Geometry: final body of the model. Coordinates: model frame, mm. Give positions to 0.01 mm unless a question says otherwise; leave off trailing zeros. Write each loop counter-clockwise with the first axis right and the second up, starting at its lowest first coordinate (ties: lowest second). Pieces come first, ordered by that corner, then holes. Notation, with made-up numbers: M 71,32 L 75,32 A11 ccw 75,49 Z; hole C 14.25,66 d3. An arc over 180 degrees is marked long. Use a Markdown table: item, result. Add a question column.
(1) Draft query along X for faces 1 (the flat face through (36, 0, -3)), 2 (the flat face through (0, 3, -3)), 3 (the cylindrical face through (1.735, 2.958, -2.194)). Return one class per face: released by +X, released by -X, zero draft, split by the parting line, or undercut.
(2) Material intervals for L1, parallel to Y at x = 9, z = -3.4; L2, parallel to Z at x = 3, y = 2.7; L3, parallel to X at y = 3, z = -3.8, sorted ascending.
(3) Cut plane A-A (y = 3). Output: boundary loops of the cut face in (x, z), plus the area to 3 significant figures.
(4) Cut plane B-B (z = -3.5). Output: boundary loops of the cut face in (x, y).
(5) Cut plane C-C (x = 70). Output: boundary loops of the cut face in (y, z).
Autodesk Inventor part; units mm, degrees
ref_plane "YZ Plane" through (0, 0, 0) normal (1, 0, 0) x (0, 1, 0)
ref_plane "XZ Plane" through (0, 0, 0) normal (0, 1, 0) x (-1, 0, 0)
ref_plane "XY Plane" through (0, 0, 0) normal (0, 0, 1) x (1, 0, 0)
sketch "Sketch1" plane through (0, 0, 0) normal (1, 0, 0) x (0, 1, 0)
  line L0 (0, 0) -> (6, 0)
  line L1 (6, 0) -> (6, -6)
  line L2 (6, -6) -> (0, -6)
  line L3 (0, -6) -> (0, 0)
  dimension "d0" = 6
  dimension "d1" = 6
extrude "Extrusion1" add sketch "Sketch1" along normal blind 73
sketch "Sketch2" plane through (0, 6, 0) normal (0, 1, 0) x (1, 0, 0)
  line L0 (0, 6) -> (73, 6) construction
  line L1 (36.5, 6) -> (36.5, 0)
  line L2 (0, 0) -> (73, 0) construction
  line L3 (0, 6) -> (0, 0) construction
  line L4 (0, 3) -> (73, 3)
  line L5 (73, 0) -> (73, 6) construction
  point P0 (3, 3)
  point P1 (70, 3)
  dimension "d8" = 3
hole "Hole1" at (3, 6, -3) at (70, 6, -3) direction (0, -1, 0) diameter 3 end through all
sketch "Sketch3" plane through (0, 0, -6) normal (0, 0, -1) x (-1, 0, 0)
  line L0 (0, 6) -> (0, 0) construction
  line L1 (0, 6) -> (-73, 6) construction
  line L2 (-73, 0) -> (-73, 6) construction
  line L3 (0, 0) -> (-73, 0) construction
  line L4 (0, 3) -> (-73, 3) construction
  line L5 (0, 6) -> (-73, 6) construction
  line L6 (-36.5, 6) -> (-36.5, 0) construction
  line L7 (0, 0) -> (-73, 0) construction
  point P0 (-9, 3)
  point P1 (-64, 3)
  dimension "d16" = 9
hole "Hole2" at (9, 3, -6) at (64, 3, -6) direction (0, 0, 1) diameter 3 end through all
equation "\"d1\" = d0"
properties part number "transverse" material "Aluminum"
Answer list:
| question | item | result |
|---|---|---|
| 1 | face 1 | zero draft |
| 1 | face 2 | released by -X |
| 1 | face 3 | undercut |
| 2 | L1 | 0 to 1.5, 4.5 to 6 |
| 2 | L2 | -6 to -4.5, -1.5 to 0 |
| 2 | L3 | 0 to 1.73, 4.27 to 7.5, 10.5 to 62.5, 65.5 to 68.73, 71.27 to 73 |
| 3 | outline | M 0,-6 L 7.5,-6 L 7.5,0 L 0,0 Z; M 10.5,-6 L 62.5,-6 L 62.5,0 L 10.5,0 Z; M 65.5,-6 L 73,-6 L 73,0 L 65.5,0 Z; hole C 3,-3 d3; hole C 70,-3 d3 |
| 3 | area | 388 mm² |
| 4 | outline | M 0,0 L 1.59,0 L 1.59,6 L 0,6 Z; M 4.41,0 L 68.59,0 L 68.59,6 L 4.41,6 Z; M 71.41,0 L 73,0 L 73,6 L 71.41,6 Z; hole C 9,3 d3; hole C 64,3 d3 |
| 5 | outline | M 0,-6 L 6,-6 L 6,-4.5 L 0,-4.5 Z; M 0,-1.5 L 6,-1.5 L 6,0 L 0,0 Z |
